Model file for the job. Use its own axes, mm. A direction names the side the tool comes from. Round coordinates to 2 decimals unless told otherwise and drop trailing zeros. Order: outer loops, then holes, each group sorted by start corner. A loop starts at its lowest first (then second) coordinate and runs counter-clockwise, first axis right, second up. Notation, with made-up numbers: M 76.25,53 L 133.25,53 A13 cw 133.25,78 Z; hole C 85,49 d5. An arc over 180 degrees is marked long. Return JSON: item names as keys, results as strings. Group by question number.
Item 1: Which spindle directions (+Z, -Z, +X, -X, +Y, -Y) get a long thin tool onto all of the face, cutting with end or side? Do faces 5 (the face through (-4.13, 44, 11)), 6 (the face through (-8.465, 8.646, 11.479)), 7 (the face through (-33.345, 5.116, 17.553)). Say none if no direction does.
Item 2: Slice it at D-D on z = 20.75. Write the cut outline in (x, y).
Item 3: Probe line 1 along Y through (x, z) = (-22.5, 10.75); line 2 along Z through (x, y) = (-38, 18); line 3 along Y through (x, z) = (-14.5, 12). List the from-to ranges inside material, lowest first.
Item 4: Slice it at C-C on x = -35. Write the cut outline in (y, z), then the cut area to 3 significant figures.
Item 5: Slice it at B-B on x = -24. Write the cut outline in (y, z), then the cut area to 3 significant figures.
Item 6: Slice it at A-A on y = 21.5. Write the cut outline in (x, z).
Item 7: Pin check, flat tips, straight feed: pin 1 Ø6 at (x, z) = (-4, 19) entering from -Y; pin 2 Ø3.5 at (x, z) = (3, 11.5) entering from +Y; pin 3 Ø0.9 at (y, z) = (44.5, 11) entering from -X. Stop position of each tip, or through.
Item 8: Pull direction Y, two halves, no side cores. Call faces 1 (the face through (-8.646, 33.395, 11.479)), 2 (the face through (-40, 39.9, 11.5)), 3 (the face through (-37.83, 21, 11)), 4 (the face through (-37.73, 44, 11)): pulls with the +Y half, pulls with the -Y half, needs draft (parallel to the pull), parting line crosses it, or undercut.
Autodesk Inventor part; units mm, degrees
ref_plane "Work Plane2" through (-40.9959, 0.8639, 22.2359) normal (0, 0, 1) x (1, 0, 0)
ref_plane "YZ Plane" through (0, 0, 0) normal (1, 0, 0) x (0, 1, 0)
ref_plane "XZ Plane" through (0, 0, 0) normal (0, 1, 0) x (-1, 0, 0)
ref_plane "Work Plane1" through (0, 0, 10) normal (0, 0, 1) x (1, 0, 0)
sketch "Sketch1" plane through (0, 0, 10) normal (0, 0, 1) x (1, 0, 0)
  line L0 (-4.0299, -0.3538) -> (-2.2322, 1.4439) construction
  arc A0 (-1.4439, 2.2322) -> (-2.2322, 1.4439) centre (-0.9299, 0.9299) ccw construction
  line L1 (-1.4439, 2.2322) -> (0.3538, 4.0299) construction
  line L2 (-37.8299, 42.8299) -> (-37.8299, 37.8299) construction
  line L3 (-37.8299, 37.8299) -> (-42.9208, 37.8299) construction
  line L4 (-37.8299, 42.2137) -> (-37.8299, 45.8299) construction
  line L5 (-37.8299, 45.8299) -> (-4.0299, 45.8299) construction
  line L6 (-4.0299, 45.8299) -> (-4.0299, 42.2137) construction
  line L7 (-4.0299, 4.0299) -> (0.3538, 4.0299)
  circle A1 centre (-20.9299, 20.9299) radius 17.5
  line L8 (-20.9299, 58.9723) -> (17.1124, 20.9299) construction
  line L9 (17.1124, 20.9299) -> (-20.9299, -17.1124) construction
  line L10 (-20.9299, -17.1124) -> (-58.9723, 20.9299) construction
  line L11 (-58.9723, 20.9299) -> (-20.9299, 58.9723) construction
  line L12 (-20.9299, 58.9723) -> (-20.9299, -17.1124) construction
  line L13 (17.1124, 20.9299) -> (-58.9723, 20.9299) construction
  line L14 (-20.9299, 58.9723) -> (32.8701, 58.9723) construction
  line L15 (-43.4299, 43.4299) -> (1.5701, 43.4299) construction
  line L16 (1.5701, 43.4299) -> (1.5701, -1.5701) construction
  line L17 (1.5701, -1.5701) -> (-43.4299, -1.5701) construction
  line L18 (-43.4299, -1.5701) -> (-43.4299, 43.4299) construction
  line L19 (-43.4299, 43.4299) -> (1.5701, -1.5701) construction
  line L20 (1.5701, 43.4299) -> (-43.4299, -1.5701) construction
  line L21 (-43.4299, 5.3876) -> (-43.4299, 36.4723)
  line L22 (-43.4299, 36.4723) -> (-36.4723, 43.4299)
  line L23 (-36.4723, 43.4299) -> (-5.3876, 43.4299)
  line L24 (-5.3876, 43.4299) -> (1.5701, 36.4723)
  line L25 (1.5701, 36.4723) -> (1.5701, 5.3876)
  line L26 (1.5701, 5.3876) -> (-5.3876, -1.5701)
  line L27 (-5.3876, -1.5701) -> (-36.4723, -1.5701)
  line L28 (-36.4723, -1.5701) -> (-43.4299, 5.3876)
  line L29 (-4.0299, 42.2137) -> (-37.8299, 42.2137)
  line L30 (-4.0299, -0.3538) -> (-4.0299, 4.0299)
  point P0 (-37.8299, 4.0299)
  point P1 (-20.9299, 20.9299)
  dimension "d18" = 53.8
  dimension "d19" = 45
  dimension "d20" = 53.8
  dimension "d21" = 45
  dimension "d22" = 45
extrude "Extrusion1" add sketch "Sketch1" along normal blind 3
sketch "Sketch2" plane through (0, 0, 13) normal (0, 0, 1) x (1, 0, 0)
  circle A0 centre (-35.9299, 35.9299) radius 3.0099 construction
  circle A1 centre (-5.93, 35.9299) radius 3.0099 construction
  circle A2 centre (-5.93, 5.93) radius 3.0099 construction
  circle A3 centre (-35.9299, 5.93) radius 3.0099 construction
  circle A4 centre (-35.9299, 35.9299) radius 2.7099
  circle A5 centre (-5.93, 35.9299) radius 2.7099
  circle A6 centre (-5.93, 5.93) radius 2.7099
  circle A7 centre (-35.9299, 5.93) radius 2.7099
  point P0 (0, 0)
  dimension "d_1" = 0.3
  dimension "d13" = 0.3
  dimension "d14" = 0.3
  dimension "d15" = 0.3
ref_plane "Work Plane2" through (-40.9959, 0.8639, 22.2359) normal (0, 0, 1) x (1, 0, 0)
extrude "Extrusion2" add sketch "Sketch2" along normal up to surface (9.2359 mm away)
sketch "Sketch3" plane through (0, 0, 10) normal (0, 0, -1) x (-1, 0, 0)
  line L0 (37.8299, -0.4701) -> (37.8299, 4.0299) construction
  line L1 (4.0299, 4.0299) -> (4.0299, -0.4701) construction
  line L2 (37.8299, -0.4701) -> (37.8299, 1.1886) construction
  line L3 (4.0299, -3.9701) -> (4.0299, -0.3538) construction
  line L4 (45.8299, 4.0299) -> (42.2137, 4.0299) construction
  line L5 (-0.3538, 4.0299) -> (-3.9701, 4.0299) construction
  line L6 (-3.9701, 37.8299) -> (-0.3538, 37.8299) construction
  line L7 (4.0299, 42.2137) -> (4.0299, 45.8299) construction
  line L8 (37.8299, 45.8299) -> (37.8299, 42.2137) construction
  line L9 (42.2137, 37.8299) -> (45.8299, 37.8299) construction
  line L10 (37.8299, 37.7299) -> (45.8299, 37.7299)
  line L11 (45.8299, 37.7299) -> (45.8299, 4.1299)
  line L12 (45.8299, 4.1299) -> (37.8299, 4.1299)
  line L13 (37.8299, 4.1299) -> (37.8299, 37.7299)
  line L14 (37.7299, 4.0299) -> (4.1299, 4.0299)
  line L15 (4.1299, 4.0299) -> (4.1299, -3.9701)
  line L16 (4.1299, -3.9701) -> (37.7299, -3.9701)
  line L17 (37.7299, -3.9701) -> (37.7299, 4.0299)
  line L18 (4.0299, 4.1299) -> (-3.9701, 4.1299)
  line L19 (-3.9701, 4.1299) -> (-3.9701, 37.7299)
  line L20 (-3.9701, 37.7299) -> (4.0299, 37.7299)
  line L21 (4.0299, 37.7299) -> (4.0299, 4.1299)
  line L22 (4.1299, 37.8299) -> (37.7299, 37.8299)
  line L23 (37.7299, 37.8299) -> (37.7299, 45.8299)
  line L24 (37.7299, 45.8299) -> (4.1299, 45.8299)
  line L25 (4.1299, 45.8299) -> (4.1299, 37.8299)
  point P0 (0, 0)
  dimension "d23" = 0.1
  dimension "d24" = 0.1
  dimension "d25" = 0.1
  dimension "d26" = 0.1
  dimension "d27" = 0.1
extrude "Extrusion3" add sketch "Sketch3" against normal up to surface (3 mm away)
equation "\"d13\" = d_1"
equation "\"d14\" = d_1"
equation "\"d15\" = d_1"
properties part number "50_Cube_Insert_Thorlabs"
Output values:
{
 "1": {"face 5": "+Z, -Z, +X, +Y", "face 6": "+Z, -Z", "face 7": "+Z"},
 "2": {"outline": "C -35.93,5.93 d5.42; C -35.93,35.93 d5.42; C -5.93,5.93 d5.42; C -5.93,35.93 d5.42"},
 "3": {"line 1": "-3.97 to 4.03, 37.83 to 45.83", "line 2": "10 to 13", "line 3": "-3.97 to 4.65, 37.21 to 45.83"},
 "4": {"outline": "M -3.97,10 L 10.52,10 L 10.52,13 L 8.48,13 L 8.48,22.24 L 3.38,22.24 L 3.38,13 L -3.97,13 Z; M 31.34,10 L 45.83,10 L 45.83,13 L 38.48,13 L 38.48,22.24 L 33.38,22.24 L 33.38,13 L 31.34,13 Z", "area": "181 mm²"},
 "5": {"outline": "M -3.97,10 L 4.03,10 L 4.03,13 L -3.97,13 Z; M 37.83,10 L 45.83,10 L 45.83,13 L 37.83,13 Z", "area": "48.0 mm²"},
 "6": {"outline": "M -45.83,10 L -37.83,10 L -37.83,13 L -45.83,13 Z; M -4.03,10 L 3.97,10 L 3.97,13 L -4.03,13 Z"},
 "7": {"pin 1": "y = 3.22", "pin 2": "y = 37.73", "pin 3": "x = -37.73"},
 "8": {"face 1": "undercut", "face 2": "pulls with the +Y half", "face 3": "undercut", "face 4": "needs draft"}
}
